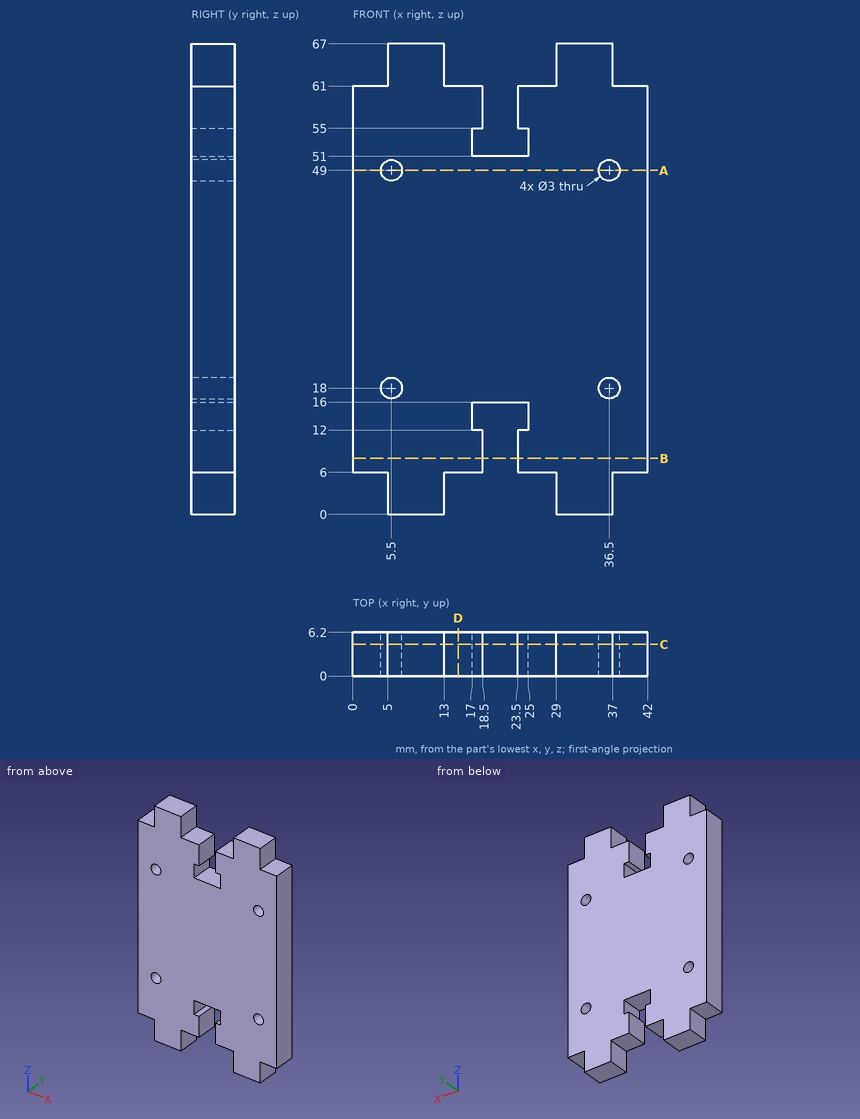
Verification items for this drawing (mm, ordinates from the low corner). Give positions to 0.01 mm unless a question says otherwise; leave off trailing zeros. Loops run counter-clockwise (first coordinate to the right, second up) from the corner with the lowest first, then second, coordinate; pieces in that order, holes last. Notation, with made-up numbers: M -11,80 L -5,80 A27 ccw -5,97 Z; hole C -37.75,-15 d7. An arc over 180 degrees is marked long. Write each question's results on one line, items separated by ' | '.
1) Section check C-C, the plane y = 4.5. Count the separate pieces of the cut face and the enclosed holes in it, plus the area to 3 significant figures.
Answers follow:
separate pieces: 1 | enclosed holes: 4 | area: 2,350 mm2
2) Section check D-D, the plane x = 15. Record the boundary of the cut face in (y, z).
Answers follow:
outline: M 0,6 L 6.2,6 L 6.2,61 L 0,61 Z
3) Thickness scan on line 1 (X direction, y = 1.75, z = 49); line 2 (X direction, y = 3.25, z = 56); line 3 (X direction, y = 2.75, z = 13.5). Record the ranges inside material, lowest first.
Answers follow:
line 1: 0 to 4, 7 to 35, 38 to 42 | line 2: 0 to 18.5, 23.5 to 42 | line 3: 0 to 17, 25 to 42
4) Section check A-A, the plane z = 49. Record the boundary of the cut face in (x, y).
Answers follow:
outline: M 0,0 L 4,0 L 4,6.2 L 0,6.2 Z; M 7,0 L 35,0 L 35,6.2 L 7,6.2 Z; M 38,0 L 42,0 L 42,6.2 L 38,6.2 Z
5) Gauge pin test, flat ends, axial feed: pin 1 (3 mm diameter, centred on x = 19, y = 2.5, fed in from +Z); pin 2 (3 mm diameter, centred on y = 3, z = 65.5, fed in from +X). Record the tip position at first contact, or that the pin passes through.
Answers follow:
pin 1: z = 61 | pin 2: x = 37
6) Section check B-B, the plane z = 8. Record the boundary of the cut face in (x, y).
Answers follow:
outline: M 0,0 L 18.5,0 L 18.5,6.2 L 0,6.2 Z; M 23.5,0 L 42,0 L 42,6.2 L 23.5,6.2 Z
